Build history of the part. All positions in model axes, mm. Round coordinates to 2 decimals unless told otherwise and drop trailing zeros. Write each loop counter-clockwise with the first axis right and the second up, starting at its lowest first coordinate (ties: lowest second). Pieces come first, ordered by that corner, then holes. Notation, with made-up numbers: M -38.5,46.5 L -32.5,46.5 A38 ccw -32.5,84.5 Z; hole C -23,-7.75 d3. An arc over 180 degrees is marked long. Use a Markdown table: item, result.
from build123d import *

# Parameters (mm, degrees)
BASE_DEPTH                = 5
ESQUISSE3_R               = 2
ESQUISSE3_W               = 65
ESQUISSE3_H               = 30
ENL_V_MAT_EXTRU_1_DEPTH   = 6
CONG_1_R                  = 3
PER_AGE_POUR_BILLES_REACH = 7
ESQUISSE6_R               = 2
ESQUISSE6_R_2             = 11
PER_AGE_POUR_PROFIL_REACH = 7
ESQUISSE8_R               = 3
ESQUISSE10_R              = 2
ENL_V_MAT_EXTRU_3_DEPTH   = 6
ESQUISSE13_R              = 2
ENL_V_MAT_EXTRU_4_DEPTH   = 10


with BuildPart() as part:
    # Esquisse1 → Base (new body)
    with BuildSketch(Plane.XY):
        Polygon((0, 0), (-175, 0), (-199.748737342, 24.748737342), (-199.748737342, 244.748737342), (-175, 269.497474683), (0, 269.497474683), (24.748737342, 244.748737342), (24.748737342, 24.748737342), align=None)
    extrude(amount=BASE_DEPTH)

    # Esquisse3 → Enlèv. mat.-Extru.1 (cut, through all)
    with BuildSketch(Plane(origin=(0, 0, 0), x_dir=(-1, 0, 0), z_dir=(0, 0, -1))):
        with Locations((52.5, 45)):
            Circle(ESQUISSE3_R)
        with Locations((122.5, 45)):
            Circle(ESQUISSE3_R)
        with Locations((122.5, 224.497474683)):
            Circle(ESQUISSE3_R)
        with Locations((52.5, 224.497474683)):
            Circle(ESQUISSE3_R)
        Polygon((129.5, 0), (129.5, 20), (105.5, 20), (105.5, 45.5), (69.5, 45.5), (69.5, 20), (45.5, 20), (45.5, 0), align=None)
        Polygon((45.5, 269.497474683), (129.5, 269.497474683), (129.5, 249.497474683), (105.5, 249.497474683), (105.5, 223.997474683), (69.5, 223.997474683), (69.5, 249.497474683), (45.5, 249.497474683), align=None)
        with Locations((87.5, 199.497474683)):
            Rectangle(ESQUISSE3_W, ESQUISSE3_H)
        with Locations((87.5, 70)):
            Rectangle(ESQUISSE3_W, ESQUISSE3_H)
    extrude(amount=-ENL_V_MAT_EXTRU_1_DEPTH, mode=Mode.SUBTRACT)

    # Congé1
    cong_1_edges = [part.edges().sort_by_distance(p)[0] for p in [
        (0, 0, 2.5),
        (-175, 0, 2.5),
        (-199.748737342, 24.748737342, 2.5),
        (-199.748737342, 244.748737342, 2.5),
        (-175, 269.497474683, 2.5),
        (0, 269.497474683, 2.5),
        (24.748737342, 244.748737342, 2.5),
        (24.748737342, 24.748737342, 2.5),
        (-45.5, 249.497474683, 2.5),
        (-45.5, 269.497474683, 2.5),
        (-129.5, 269.497474683, 2.5),
        (-129.5, 249.497474683, 2.5),
        (-105.5, 249.497474683, 2.5),
        (-105.5, 223.997474683, 2.5),
        (-69.5, 223.997474683, 2.5),
        (-69.5, 249.497474683, 2.5),
        (-129.5, 0, 2.5),
        (-45.5, 0, 2.5),
        (-45.5, 20, 2.5),
        (-69.5, 20, 2.5),
        (-69.5, 45.5, 2.5),
        (-105.5, 45.5, 2.5),
        (-105.5, 20, 2.5),
        (-129.5, 20, 2.5),
    ]]
    fillet(cong_1_edges, radius=CONG_1_R)

    # Esquisse6 → Perçage pour billes (cut, up to next)
    with BuildSketch(Plane.XY.offset(5), mode=Mode.PRIVATE) as per_age_pour_billes_sk1:
        with Locations((-12.390872965, 15.893398282)):
            Circle(ESQUISSE6_R)
    per_age_pour_billes_tool1 = extrude(per_age_pour_billes_sk1.sketch, amount=-PER_AGE_POUR_BILLES_REACH, mode=Mode.PRIVATE) & part.part
    add(per_age_pour_billes_tool1.solids().sort_by_distance((-12.390873, 15.893398, 5))[0], mode=Mode.SUBTRACT)
    # Esquisse6 → Perçage pour billes (cut, up to next)
    with BuildSketch(Plane.XY.offset(5), mode=Mode.PRIVATE) as per_age_pour_billes_sk2:
        with Locations((8.82233047, 37.106601718)):
            Circle(ESQUISSE6_R)
    per_age_pour_billes_tool2 = extrude(per_age_pour_billes_sk2.sketch, amount=-PER_AGE_POUR_BILLES_REACH, mode=Mode.PRIVATE) & part.part
    add(per_age_pour_billes_tool2.solids().sort_by_distance((8.82233, 37.106602, 5))[0], mode=Mode.SUBTRACT)
    # Esquisse6 → Perçage pour billes (cut, up to next)
    with BuildSketch(Plane.XY.offset(5), mode=Mode.PRIVATE) as per_age_pour_billes_sk3:
        with Locations((8.82233047, 232.390872965)):
            Circle(ESQUISSE6_R)
    per_age_pour_billes_tool3 = extrude(per_age_pour_billes_sk3.sketch, amount=-PER_AGE_POUR_BILLES_REACH, mode=Mode.PRIVATE) & part.part
    add(per_age_pour_billes_tool3.solids().sort_by_distance((8.82233, 232.390873, 5))[0], mode=Mode.SUBTRACT)
    # Esquisse6 → Perçage pour billes (cut, up to next)
    with BuildSketch(Plane.XY.offset(5), mode=Mode.PRIVATE) as per_age_pour_billes_sk4:
        with Locations((-12.390872965, 253.604076401)):
            Circle(ESQUISSE6_R)
    per_age_pour_billes_tool4 = extrude(per_age_pour_billes_sk4.sketch, amount=-PER_AGE_POUR_BILLES_REACH, mode=Mode.PRIVATE) & part.part
    add(per_age_pour_billes_tool4.solids().sort_by_distance((-12.390873, 253.604076, 5))[0], mode=Mode.SUBTRACT)
    # Esquisse6 → Perçage pour billes (cut, up to next)
    with BuildSketch(Plane.XY.offset(5), mode=Mode.PRIVATE) as per_age_pour_billes_sk5:
        with Locations((-1.784271247, 242.997474683)):
            Circle(ESQUISSE6_R_2)
    per_age_pour_billes_tool5 = extrude(per_age_pour_billes_sk5.sketch, amount=-PER_AGE_POUR_BILLES_REACH, mode=Mode.PRIVATE) & part.part
    add(per_age_pour_billes_tool5.solids().sort_by_distance((-1.784271, 242.997475, 5))[0], mode=Mode.SUBTRACT)
    # Esquisse6 → Perçage pour billes (cut, up to next)
    with BuildSketch(Plane.XY.offset(5), mode=Mode.PRIVATE) as per_age_pour_billes_sk6:
        with Locations((-1.784271247, 26.5)):
            Circle(ESQUISSE6_R_2)
    per_age_pour_billes_tool6 = extrude(per_age_pour_billes_sk6.sketch, amount=-PER_AGE_POUR_BILLES_REACH, mode=Mode.PRIVATE) & part.part
    add(per_age_pour_billes_tool6.solids().sort_by_distance((-1.784271, 26.5, 5))[0], mode=Mode.SUBTRACT)
    # Esquisse6 → Perçage pour billes (cut, up to next)
    with BuildSketch(Plane.XY.offset(5), mode=Mode.PRIVATE) as per_age_pour_billes_sk7:
        with Locations((-144.142135624, 190.104076401)):
            Circle(ESQUISSE6_R)
    per_age_pour_billes_tool7 = extrude(per_age_pour_billes_sk7.sketch, amount=-PER_AGE_POUR_BILLES_REACH, mode=Mode.PRIVATE) & part.part
    add(per_age_pour_billes_tool7.solids().sort_by_distance((-144.142136, 190.104076, 5))[0], mode=Mode.SUBTRACT)
    # Esquisse6 → Perçage pour billes (cut, up to next)
    with BuildSketch(Plane.XY.offset(5), mode=Mode.PRIVATE) as per_age_pour_billes_sk8:
        with Locations((-165.355339059, 168.890872965)):
            Circle(ESQUISSE6_R)
    per_age_pour_billes_tool8 = extrude(per_age_pour_billes_sk8.sketch, amount=-PER_AGE_POUR_BILLES_REACH, mode=Mode.PRIVATE) & part.part
    add(per_age_pour_billes_tool8.solids().sort_by_distance((-165.355339, 168.890873, 5))[0], mode=Mode.SUBTRACT)
    # Esquisse6 → Perçage pour billes (cut, up to next)
    with BuildSketch(Plane.XY.offset(5), mode=Mode.PRIVATE) as per_age_pour_billes_sk9:
        with Locations((-154.748737342, 179.497474683)):
            Circle(ESQUISSE6_R_2)
    per_age_pour_billes_tool9 = extrude(per_age_pour_billes_sk9.sketch, amount=-PER_AGE_POUR_BILLES_REACH, mode=Mode.PRIVATE) & part.part
    add(per_age_pour_billes_tool9.solids().sort_by_distance((-154.748737, 179.497475, 5))[0], mode=Mode.SUBTRACT)
    # Esquisse6 → Perçage pour billes (cut, up to next)
    with BuildSketch(Plane.XY.offset(5), mode=Mode.PRIVATE) as per_age_pour_billes_sk10:
        with Locations((-165.355339059, 100.606601718)):
            Circle(ESQUISSE6_R)
    per_age_pour_billes_tool10 = extrude(per_age_pour_billes_sk10.sketch, amount=-PER_AGE_POUR_BILLES_REACH, mode=Mode.PRIVATE) & part.part
    add(per_age_pour_billes_tool10.solids().sort_by_distance((-165.355339, 100.606602, 5))[0], mode=Mode.SUBTRACT)
    # Esquisse6 → Perçage pour billes (cut, up to next)
    with BuildSketch(Plane.XY.offset(5), mode=Mode.PRIVATE) as per_age_pour_billes_sk11:
        with Locations((-154.748737342, 90)):
            Circle(ESQUISSE6_R_2)
    per_age_pour_billes_tool11 = extrude(per_age_pour_billes_sk11.sketch, amount=-PER_AGE_POUR_BILLES_REACH, mode=Mode.PRIVATE) & part.part
    add(per_age_pour_billes_tool11.solids().sort_by_distance((-154.748737, 90, 5))[0], mode=Mode.SUBTRACT)
    # Esquisse6 → Perçage pour billes (cut, up to next)
    with BuildSketch(Plane.XY.offset(5), mode=Mode.PRIVATE) as per_age_pour_billes_sk12:
        with Locations((-144.142135624, 79.393398282)):
            Circle(ESQUISSE6_R)
    per_age_pour_billes_tool12 = extrude(per_age_pour_billes_sk12.sketch, amount=-PER_AGE_POUR_BILLES_REACH, mode=Mode.PRIVATE) & part.part
    add(per_age_pour_billes_tool12.solids().sort_by_distance((-144.142136, 79.393398, 5))[0], mode=Mode.SUBTRACT)
    # Esquisse6 → Perçage pour billes (cut, up to next)
    with BuildSketch(Plane.XY.offset(5), mode=Mode.PRIVATE) as per_age_pour_billes_sk13:
        with Locations((-183.838834765, 37.123106012)):
            Circle(ESQUISSE6_R)
    per_age_pour_billes_tool13 = extrude(per_age_pour_billes_sk13.sketch, amount=-PER_AGE_POUR_BILLES_REACH, mode=Mode.PRIVATE) & part.part
    add(per_age_pour_billes_tool13.solids().sort_by_distance((-183.838835, 37.123106, 5))[0], mode=Mode.SUBTRACT)
    # Esquisse6 → Perçage pour billes (cut, up to next)
    with BuildSketch(Plane.XY.offset(5), mode=Mode.PRIVATE) as per_age_pour_billes_sk14:
        with Locations((-162.625631329, 15.909902577)):
            Circle(ESQUISSE6_R)
    per_age_pour_billes_tool14 = extrude(per_age_pour_billes_sk14.sketch, amount=-PER_AGE_POUR_BILLES_REACH, mode=Mode.PRIVATE) & part.part
    add(per_age_pour_billes_tool14.solids().sort_by_distance((-162.625631, 15.909903, 5))[0], mode=Mode.SUBTRACT)
    # Esquisse6 → Perçage pour billes (cut, up to next)
    with BuildSketch(Plane.XY.offset(5), mode=Mode.PRIVATE) as per_age_pour_billes_sk15:
        with Locations((-162.625631329, 253.587572106)):
            Circle(ESQUISSE6_R)
    per_age_pour_billes_tool15 = extrude(per_age_pour_billes_sk15.sketch, amount=-PER_AGE_POUR_BILLES_REACH, mode=Mode.PRIVATE) & part.part
    add(per_age_pour_billes_tool15.solids().sort_by_distance((-162.625631, 253.587572, 5))[0], mode=Mode.SUBTRACT)
    # Esquisse6 → Perçage pour billes (cut, up to next)
    with BuildSketch(Plane.XY.offset(5), mode=Mode.PRIVATE) as per_age_pour_billes_sk16:
        with Locations((-183.838834765, 232.374368671)):
            Circle(ESQUISSE6_R)
    per_age_pour_billes_tool16 = extrude(per_age_pour_billes_sk16.sketch, amount=-PER_AGE_POUR_BILLES_REACH, mode=Mode.PRIVATE) & part.part
    add(per_age_pour_billes_tool16.solids().sort_by_distance((-183.838835, 232.374369, 5))[0], mode=Mode.SUBTRACT)

    # Esquisse8 → Perçage pour profilé (cut, up to next)
    with BuildSketch(Plane.XY.offset(5), mode=Mode.PRIVATE) as per_age_pour_profil_sk1:
        with Locations((-142, 12.5)):
            Circle(ESQUISSE8_R)
    per_age_pour_profil_tool1 = extrude(per_age_pour_profil_sk1.sketch, amount=-PER_AGE_POUR_PROFIL_REACH, mode=Mode.PRIVATE) & part.part
    add(per_age_pour_profil_tool1.solids().sort_by_distance((-142, 12.5, 5))[0], mode=Mode.SUBTRACT)
    # Esquisse8 → Perçage pour profilé (cut, up to next)
    with BuildSketch(Plane.XY.offset(5), mode=Mode.PRIVATE) as per_age_pour_profil_sk2:
        with Locations((-142, 256.997474683)):
            Circle(ESQUISSE8_R)
    per_age_pour_profil_tool2 = extrude(per_age_pour_profil_sk2.sketch, amount=-PER_AGE_POUR_PROFIL_REACH, mode=Mode.PRIVATE) & part.part
    add(per_age_pour_profil_tool2.solids().sort_by_distance((-142, 256.997475, 5))[0], mode=Mode.SUBTRACT)
    # Esquisse8 → Perçage pour profilé (cut, up to next)
    with BuildSketch(Plane.XY.offset(5), mode=Mode.PRIVATE) as per_age_pour_profil_sk3:
        with Locations((-33, 256.997474683)):
            Circle(ESQUISSE8_R)
    per_age_pour_profil_tool3 = extrude(per_age_pour_profil_sk3.sketch, amount=-PER_AGE_POUR_PROFIL_REACH, mode=Mode.PRIVATE) & part.part
    add(per_age_pour_profil_tool3.solids().sort_by_distance((-33, 256.997475, 5))[0], mode=Mode.SUBTRACT)
    # Esquisse8 → Perçage pour profilé (cut, up to next)
    with BuildSketch(Plane.XY.offset(5), mode=Mode.PRIVATE) as per_age_pour_profil_sk4:
        with Locations((-33, 12.5)):
            Circle(ESQUISSE8_R)
    per_age_pour_profil_tool4 = extrude(per_age_pour_profil_sk4.sketch, amount=-PER_AGE_POUR_PROFIL_REACH, mode=Mode.PRIVATE) & part.part
    add(per_age_pour_profil_tool4.solids().sort_by_distance((-33, 12.5, 5))[0], mode=Mode.SUBTRACT)

    # Esquisse10 → Enlèv. mat.-Extru.3 (cut, through all)
    with BuildSketch(Plane.XY.offset(5)):
        with Locations((-120.5, 174.497474683)):
            Circle(ESQUISSE10_R)
        with Locations((-120.5, 147.997474683)):
            Circle(ESQUISSE10_R)
        with Locations((-54.5, 147.997474683)):
            Circle(ESQUISSE10_R)
        with Locations((-54.5, 174.497474683)):
            Circle(ESQUISSE10_R)
        with Locations((-54.5, 121.5)):
            Circle(ESQUISSE10_R)
        with Locations((-54.5, 95)):
            Circle(ESQUISSE10_R)
        with Locations((-120.5, 121.5)):
            Circle(ESQUISSE10_R)
        with Locations((-120.5, 95)):
            Circle(ESQUISSE10_R)
    extrude(amount=-ENL_V_MAT_EXTRU_3_DEPTH, mode=Mode.SUBTRACT)

    # Esquisse13 → Enlèv. mat.-Extru.4 (cut)
    with BuildSketch(Plane.XY.offset(5)):
        with Locations((-20.251262658, 184.748737342)):
            Circle(ESQUISSE13_R)
        with Locations((-20.251262658, 164.748737342)):
            Circle(ESQUISSE13_R)
        with Locations((-20.251262658, 104.748737342)):
            Circle(ESQUISSE13_R)
        with Locations((-20.251262658, 84.748737342)):
            Circle(ESQUISSE13_R)
    extrude(amount=-ENL_V_MAT_EXTRU_4_DEPTH, mode=Mode.SUBTRACT)


solid = part.part
Q1. Cut at A-A on y = 90. Give the cut face in (x, z).
Response values:
| item | result |
|---|---|
| outline | M -199.75,0 L -165.75,0 L -165.75,5 L -199.75,5 Z; M -143.75,0 L 24.75,0 L 24.75,5 L -143.75,5 Z |
Q2. Drop flat-ended pins along their axis: P1, Ø13, axis at x = -1.78, y = 243, coming from the -Z side; P2, Ø3, axis at x = -100.5, z = 4, coming from the +Y side; P3, Ø5, axis at x = -20.25, y = 104.75, coming from the +Z side; P4, Ø1.5, axis at y = 261.5, z = 2, coming from the +X side. Give the stop position or say it passes through.
Response values:
| item | result |
|---|---|
| P1 | passes through |
| P2 | stops at y = 224 |
| P3 | stops at z = 5 |
| P4 | stops at x = 8.75 |
Q3. Drill centre lines: L1, parallel to Y at x = -108.5, z = 0.45; L2, parallel to Y at x = -94.5, z = 2; L3, parallel to Y at x = -18.5, z = 0.8. Where is each one in solid material? Low to high.
Response values:
| item | result |
|---|---|
| L1 | y = 20 to 55, 85 to 184.5, 214.5 to 249.5 |
| L2 | y = 45.5 to 55, 85 to 184.5, 214.5 to 224 |
| L3 | y = 0 to 83.78, 85.71 to 103.78, 105.71 to 163.78, 165.71 to 183.78, 185.71 to 269.5 |
Q4. Cut at B-B on z = 3.9. Count the separate pieces of the cut face and the enclosed holes in it, and give its area (3 significant figures).
Response values:
| item | result |
|---|---|
| separate pieces | 1 |
| enclosed holes | 38 |
| area | 48,200 mm2 |
Q5. Two-plate mould, pull along Y, no slides. Class faces 1 (the flat face through (-86, 137, 0)), 2 (the cylindrical face through (-33.65, 254.07, 2.54)), 3 (the flat face through (12.2, 257.3, 2.5)): +Y half, -Y half, draft (parallel to the pull), parting line (faces both ways), or undercut.
Response values:
| item | result |
|---|---|
| face 1 | draft |
| face 2 | undercut |
| face 3 | +Y half |
